```python
from build123d import *

# Parameters (mm, degrees)
SKETCH1_W           = 240
SKETCH1_H           = 100
BOSS_EXTRUDE1_DEPTH = 1.6
CUT_EXTRUDE1_REACH  = 262.005
SKETCH2_R           = 2.5
LPATTERN1_COUNT     = 6
LPATTERN1_PITCH     = 15.88
CUT_EXTRUDE2_REACH  = 262.005
SKETCH3_W           = 71
SKETCH3_H           = 28
CUT_EXTRUDE3_REACH  = 262.005
SKETCH4_W           = 20
SKETCH4_H           = 20


with BuildPart() as part:
    # Sketch1 → Boss-Extrude1 (new body)
    with BuildSketch(Plane.XY):
        with Locations((120, 50)):
            Rectangle(SKETCH1_W, SKETCH1_H)
    extrude(amount=BOSS_EXTRUDE1_DEPTH)

    # Sketch2 → Cut-Extrude1 (cut, up to next)
    with BuildSketch(Plane.XY.offset(1.6), mode=Mode.PRIVATE) as cut_extrude1_sk1:
        with Locations((5.6, 10.3)):
            Circle(SKETCH2_R)
    cut_extrude1_tool1 = extrude(cut_extrude1_sk1.sketch, amount=-CUT_EXTRUDE1_REACH, mode=Mode.PRIVATE) & part.part
    # Sketch2 → Cut-Extrude1 (cut, up to next)
    with BuildSketch(Plane.XY.offset(1.6), mode=Mode.PRIVATE) as cut_extrude1_sk2:
        with Locations((234.4, 10.3)):
            Circle(SKETCH2_R)
    cut_extrude1_tool2 = extrude(cut_extrude1_sk2.sketch, amount=-CUT_EXTRUDE1_REACH, mode=Mode.PRIVATE) & part.part
    cut_extrude1_1 = cut_extrude1_tool1.solids().sort_by_distance((5.6, 10.3, 1.6))[0]
    add(cut_extrude1_1, mode=Mode.SUBTRACT)
    cut_extrude1_2 = cut_extrude1_tool2.solids().sort_by_distance((234.4, 10.3, 1.6))[0]
    add(cut_extrude1_2, mode=Mode.SUBTRACT)
    cut_extrude1 = cut_extrude1_1 + cut_extrude1_2  # Cut-Extrude1 as one shape, for the pattern or mirror that repeats it

    # LPattern1: Cut-Extrude1 ×6
    with Locations(*[(0, i * LPATTERN1_PITCH, 0) for i in range(1, LPATTERN1_COUNT)]):
        add(cut_extrude1, mode=Mode.SUBTRACT)

    # Sketch3 → Cut-Extrude2 (cut, up to next)
    with BuildSketch(Plane.XY.offset(1.6), mode=Mode.PRIVATE) as cut_extrude2_sk1:
        with Locations((52.5, 14)):
            Rectangle(SKETCH3_W, SKETCH3_H)
    cut_extrude2_tool1 = extrude(cut_extrude2_sk1.sketch, amount=-CUT_EXTRUDE2_REACH, mode=Mode.PRIVATE) & part.part
    add(cut_extrude2_tool1.solids().sort_by_distance((52.5, 14, 1.6))[0], mode=Mode.SUBTRACT)

    # Sketch4 → Cut-Extrude3 (cut, up to next)
    with BuildSketch(Plane(origin=(0, 0, 0), x_dir=(-1, 0, 0), z_dir=(0, 0, -1)), mode=Mode.PRIVATE) as cut_extrude3_sk1:
        with Locations((-210, 10)):
            Rectangle(SKETCH4_W, SKETCH4_H)
    cut_extrude3_tool1 = extrude(cut_extrude3_sk1.sketch, amount=-CUT_EXTRUDE3_REACH, mode=Mode.PRIVATE) & part.part
    add(cut_extrude3_tool1.solids().sort_by_distance((210, 10, 0))[0], mode=Mode.SUBTRACT)


solid = part.part
```
Design review of the part built by this model. Coordinates are the model's own, in mm. Coordinates: 2 decimals unless noted, no trailing zeros. Loops run counter-clockwise (first coordinate to the right, second up) from the corner with the lowest first, then second, coordinate; pieces in that order, holes last.
Q1. We need section D-D on x = 234.4. State the section outline as (y, z) points, and give its area (3 significant figures).
Reported:
outline: (0, 0) - (7.8, 0) - (7.8, 1.6) - (0, 1.6) - close; (12.8, 0) - (23.68, 0) - (23.68, 1.6) - (12.8, 1.6) - close; (28.68, 0) - (39.56, 0) - (39.56, 1.6) - (28.68, 1.6) - close; (44.56, 0) - (55.44, 0) - (55.44, 1.6) - (44.56, 1.6) - close; (60.44, 0) - (71.32, 0) - (71.32, 1.6) - (60.44, 1.6) - close; (76.32, 0) - (87.2, 0) - (87.2, 1.6) - (76.32, 1.6) - close; (92.2, 0) - (100, 0) - (100, 1.6) - (92.2, 1.6) - close
area: 112 mm2
Q2. We need section B-B on y = 10.3. State the section outline as (x, z) points, and give its area (3 significant figures).
Reported:
outline: (0, 0) - (3.1, 0) - (3.1, 1.6) - (0, 1.6) - close; (8.1, 0) - (17, 0) - (17, 1.6) - (8.1, 1.6) - close; (88, 0) - (200, 0) - (200, 1.6) - (88, 1.6) - close; (220, 0) - (231.9, 0) - (231.9, 1.6) - (220, 1.6) - close; (236.9, 0) - (240, 0) - (240, 1.6) - (236.9, 1.6) - close
area: 222 mm2
Q3. We need section A-A on z = 0.55. State how many separate pieces and enclosed holes the cut face has, and give its area (3 significant figures).
Reported:
separate pieces: 1
enclosed holes: 12
area: 21,400 mm2
Q4. The part is to be moulded in two halves that separate along X. For faces 1 (the face through (118, 51, 0)), 2 (the face through (5.06, 55.5, 0.81)), 3 (the face through (231.9, 58, 0.8)), say which applies: +X half, -X half, draft (parallel to the pull), parting line (faces both ways), or undercut.
Reported:
face 1: draft
face 2: undercut
face 3: undercut
Q5. To check wall thickness, follow line 1 (Y direction, x = 202.5, z = 0.2); line 2 (Y direction, x = 62, z = 0.7). State the ranges of each line that lie inside material, in increasing order.
Reported:
line 1: y = 20 to 100
line 2: y = 28 to 100
Q6. We need section C-C on y = 57.94. State the section outline as (x, z) points.
Reported:
outline: (0, 0) - (3.1, 0) - (3.1, 1.6) - (0, 1.6) - close; (8.1, 0) - (231.9, 0) - (231.9, 1.6) - (8.1, 1.6) - close; (236.9, 0) - (240, 0) - (240, 1.6) - (236.9, 1.6) - close
Q7. For pin 1 (0.8 mm diameter, centred on x = 214.5, z = 1, fed in from -Y), flat-tipped, find the tip position at first contact; note if it passes through.
Reported:
pin 1: stops at y = 20
